Source: CAD feature listing. Evaluate the final solid. Frame: model axes, mm. Face numbers are marked on the shaded views. A direction names the side the tool comes from. Coordinates: 2 decimals unless noted, no trailing zeros. Write each loop counter-clockwise with the first axis right and the second up, starting at its lowest first coordinate (ties: lowest second). Pieces come first, ordered by that corner, then holes. Notation, with made-up numbers: (88.25, 69) - (107.25, 69) arc R18 cw to (107.25, 74) - close; hole circle Ø5 at (-29.5, -26.75). An arc over 180 degrees is marked (long way). One line per question, with ' | ' between items.
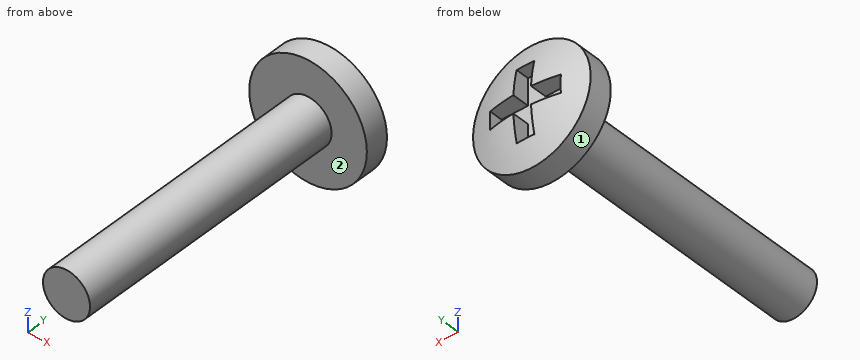
from build123d import *

# Parameters (mm, degrees)
SKETCH1_R           = 1
BOSS_EXTRUDE1_DEPTH = 12
SKETCH2_R           = 2.5
BOSS_EXTRUDE2_DEPTH = 1
DOME1_FACE_RADIUS   = 2.5
DOME1_HEIGHT        = 0.5
SKETCH3_W           = 1.125
SKETCH3_H           = 0.75
SKETCH3_W_2         = 0.75
SKETCH3_H_2         = 1.125
CUT_EXTRUDE1_DEPTH  = 0.75


with BuildPart() as part:
    # Sketch1 → Boss-Extrude1 (new body)
    with BuildSketch(Plane(origin=(0, 0, 0), x_dir=(1, 0, 0), z_dir=(0, 1, 0))):
        Circle(SKETCH1_R)
    extrude(amount=BOSS_EXTRUDE1_DEPTH)

    # Sketch2 → Boss-Extrude2 (add)
    with BuildSketch(Plane(origin=(0, 12, 0), x_dir=(1, 0, 0), z_dir=(0, 1, 0))):
        Circle(SKETCH2_R)
    extrude(amount=BOSS_EXTRUDE2_DEPTH)

    # Dome1: a dome of height H over a round flat face of radius A is a cap of a sphere of radius (A * A + H * H) / (2 * H)
    dome1_r = (DOME1_FACE_RADIUS * DOME1_FACE_RADIUS + DOME1_HEIGHT * DOME1_HEIGHT) / (2 * DOME1_HEIGHT)
    dome1_base = Plane((0, 13, 0), z_dir=(0, 1, 0))
    with Locations(dome1_base.offset(DOME1_HEIGHT - dome1_r)):
        dome1_ball = Sphere(dome1_r, mode=Mode.PRIVATE)
    add(split(dome1_ball, bisect_by=dome1_base, keep=Keep.TOP, mode=Mode.PRIVATE))

    # Sketch3 → Cut-Extrude1 (cut)
    with BuildSketch(Plane(origin=(0, 13.5, 0), x_dir=(1, 0, 0), z_dir=(0, 1, 0))):
        with Locations((-0.9375, 0)):
            Rectangle(SKETCH3_W, SKETCH3_H)
        Rectangle(SKETCH3_W_2, SKETCH3_H)
        with Locations((0, 0.9375)):
            Rectangle(SKETCH3_W_2, SKETCH3_H_2)
        with Locations((0.9375, 0)):
            Rectangle(SKETCH3_W, SKETCH3_H)
        with Locations((0, -0.9375)):
            Rectangle(SKETCH3_W_2, SKETCH3_H_2)
    extrude(amount=-CUT_EXTRUDE1_DEPTH, mode=Mode.SUBTRACT)


solid = part.part
Item 1: Cut plane A-A on x = 0. Return loops of the section in (y, z).
Check sheet entries:
outline: (0, -1) - (12, -1) - (12, -2.5) - (13, -2.5) arc R6.5 ccw to (13.32, -1.5) - (12.75, -1.5) - (12.75, 1.5) - (13.32, 1.5) arc R6.5 ccw to (13, 2.5) - (12, 2.5) - (12, 1) - (0, 1) - close
Item 2: Cut plane D-D on z = -1.15. Return loops of the section in (x, y) (3 decimals).
Check sheet entries:
outline: (-2.22, 12) - (2.22, 12) - (2.22, 13) arc R6.397 ccw to (0.375, 13.386) - (0.375, 12.75) - (-0.375, 12.75) - (-0.375, 13.386) arc R6.397 ccw to (-2.22, 13) - close
Item 3: Access query for the marked faces 1 and 2. Directions: +Z, -Z, +X, -X, +Y, -Y. A direction counts if a zero-diameter tool reaches every point of the face in a straight line with its end or side. Return the directions, or none.
Check sheet entries:
face 1: +Y, -Y | face 2: -Y
Item 4: Cut plane C-C on y = 9.5. Return loops of the section in (x, z).
Check sheet entries:
outline: circle Ø2 at (0, 0)
Item 5: Ray query, line 1 along Y through (x, z) = (0.8, 0.25); line 2 along Y through (x, z) = (-0.25, 1.1); line 3 along Z through (x, y) = (0.25, 3.5). Return the intervals inside material, ascending. Write a range as [from, to].
Check sheet entries:
line 1: [0, 12.75] | line 2: [12, 12.75] | line 3: [-0.97, 0.97]
Item 6: Pin query (flat end, axial travel): pin 1 Ø0.8 at (y, z) = (13, 1) entering from +X; pin 2 Ø1.5 at (x, z) = (-1, -1) entering from +Y; pin 3 Ø3 at (y, z) = (7, 0) entering from +X. Return the tip coordinate at first contact, or that it passes through.
Check sheet entries:
pin 1: x = 2.43 | pin 2: y = 13.47 | pin 3: x = 1
Item 7: Cut plane B-B on z = 0. Return loops of the section in (x, y).
Check sheet entries:
outline: (-2.5, 12) - (-1, 12) - (-1, 0) - (1, 0) - (1, 12) - (2.5, 12) - (2.5, 13) arc R6.5 ccw to (1.5, 13.32) - (1.5, 12.75) - (-1.5, 12.75) - (-1.5, 13.32) arc R6.5 ccw to (-2.5, 13) - close
